Part model, mm, in its own coordinate system. A direction names the side the tool comes from. Round coordinates to 2 decimals unless told otherwise and drop trailing zeros. Write each loop counter-clockwise with the first axis right and the second up, starting at its lowest first coordinate (ties: lowest second). Pieces come first, ordered by that corner, then holes.
from build123d import *

# Parameters (mm, degrees)
F0_R     = 8.5
F1_DEPTH = 4
F2_R     = 5
F3_DEPTH = 100
F5_DEPTH = 5


with BuildPart() as f1:
    # F0 (on Top) → F1 (new body)
    with BuildSketch(Plane.XY):
        Circle(F0_R)
    extrude(amount=F1_DEPTH)

    # F2 (on Top) → F3 (join)
    with BuildSketch(Plane.XY):
        Circle(F2_R)
    extrude(amount=F3_DEPTH)

    # F4 (on face) → F5 (join)
    with BuildSketch(Plane.XY.offset(100)):
        Polygon((0.674898, -0.737911), (0.976499, 0.215523), (0.301601, 0.953434), (-0.674898, 0.737911), (-0.976499, -0.215523), (-0.301601, -0.953434), align=None)
    extrude(amount=F5_DEPTH)


solid = f1.part
Q1. Saw through at A-A, the plane x = -3. Write the cut outline in (y, z).
Q2. Saw through at D-D, the plane x = 3.5. Write the cut outline in (y, z).
Q3. Wall check: line 1 (Z direction, x = -5.75, y = 1.5); line 2 (Z direction, x = 3.75, y = 0.25); line 3 (X direction, y = 0, z = 17). Give the ranges that are in metal, low to high.
Q4. Drop flat-ended pins along their axis: P1, Ø5, axis at y = 4, z = 69, coming from the +X side; P2, Ø8, axis at x = -6.5, y = 1, coming from the +Z side; P3, Ø2, axis at y = -1.5, z = 60.5, coming from the +X side. Give the stop position or say it passes through.
Q5. Saw through at C-C, the plane y = -7.25. Write the cut outline in (x, z).
Q6. Saw through at B-B, the plane z = 91.5. Write the cut outline in (x, y), and give its area (3 significant figures).
Q7. Tool access for faces 1 (the flat face through (4, -4, 4)), 2 (the flat face through (0, 0, 0)): list every direction of +Z, -Z, +X, -X, +Y, -Y with a clear straight run to the whole face (end or side of a thin tool).
Computed:
1. outline: (-7.95, 0) - (7.95, 0) - (7.95, 4) - (4, 4) - (4, 100) - (-4, 100) - (-4, 4) - (-7.95, 4) - close
2. outline: (-7.75, 0) - (7.75, 0) - (7.75, 4) - (3.57, 4) - (3.57, 100) - (-3.57, 100) - (-3.57, 4) - (-7.75, 4) - close
3. line 1: z = 0 to 4
3. line 2: z = 0 to 100
3. line 3: x = -5 to 5
4. P1: stops at x = 4.77
4. P2: stops at z = 100
4. P3: stops at x = 4.97
5. outline: (-4.44, 0) - (4.44, 0) - (4.44, 4) - (-4.44, 4) - close
6. outline: circle Ø10 at (0, 0)
6. area: 78.5 mm2
7. face 1: +Z
7. face 2: -Z, +X, -X, +Y, -Y
